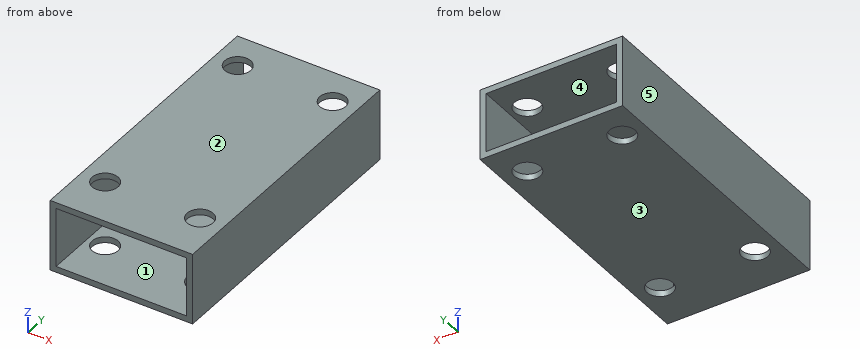
from build123d import *

# Parameters (mm, degrees)
SKETCH1_W               = 76.2
SKETCH1_H               = 38.1
EXTRUDE1_DEPTH          = 76.2
SKETCH2_W               = 69.85
SKETCH2_H               = 31.75
EXTRUDE2_DEPTH          = 159.241184589
F_1_2_CLEARANCE_HOLE1_D = 13.89126


with BuildPart() as part:
    # Sketch1 → Extrude1 (new, symmetric)
    with BuildSketch(Plane(origin=(0, 0, 0), x_dir=(1, 0, 0), z_dir=(0, 1, 0))):
        Rectangle(SKETCH1_W, SKETCH1_H)
    extrude(amount=EXTRUDE1_DEPTH, both=True)

    # Sketch2 → Extrude2 (cut, through all)
    with BuildSketch(Plane(origin=(0, 76.2, 0), x_dir=(1, 0, 0), z_dir=(0, 1, 0))):
        Rectangle(SKETCH2_W, SKETCH2_H)
    extrude(amount=-EXTRUDE2_DEPTH, mode=Mode.SUBTRACT)

    # 1/2 Clearance Hole1 (through all)
    with Locations(Plane.XY.offset(19.05)):
        with Locations((25.4, 57.15), (-25.4, 57.15), (-25.4, -50.8), (25.4, -50.8)):
            Hole(F_1_2_CLEARANCE_HOLE1_D / 2)


solid = part.part
Could you check a few things on this model? Use its own coordinates, in mm. Face numbers are marked on the shaded views. A direction names the side the tool comes from. Give positions to 0.01 mm unless a question says otherwise; leave off trailing zeros. Order: outer loops, then holes, each group sorted by start corner. A loop starts at its lowest first (then second) coordinate and runs counter-clockwise, first axis right, second up.
1. Suppose I cut it at D-D (y = 45.5). List the corners of the cut face in (x, z) for me (3 decimals), plus the area to 3 significant figures.
2. For the marked faces 1 and 2, which set-ups out of +Z, -Z, +X, -X, +Y, -Y let a thin tool reach every point of the face, with its end or its side?
3. I need wall thicknesses on L1, parallel to Y at x = -25, z = -17; L2, parallel to X at y = 57, z = 16; L3, parallel to Z at x = 9.5, y = 7.5 (3 decimals). Which ranges of each line are inside material? Lowest first, please.
4. Will this pin go through, and if not, where does the flat tip stop? P1, Ø18, axis at x = -25.4, y = 57.15, coming from the -Z side.
5. Suppose I cut it at A-A (z = -9). List the corners of the cut face in (x, y) for me (3 decimals), plus the area to 3 significant figures.
6. Suppose I cut it at B-B (x = 25.4). List the corners of the cut face in (y, z) for me (3 decimals), plus the area to 3 significant figures.
7. We'd pull the mould along Z, two halves only. Please class the marked faces 3, 4 and 5: pulls with the +Z half, pulls with the -Z half, needs draft (parallel to the pull), parting line crosses it, or undercut.
8. Suppose I cut it at C-C (y = -47.5). List the corners of the cut face in (x, z) for me (3 decimals), plus the area to 3 significant figures.
Solved:
1. outline: (-38.1, -19.05) - (38.1, -19.05) - (38.1, 19.05) - (-38.1, 19.05) - close; hole (-34.925, -15.875) - (34.925, -15.875) - (34.925, 15.875) - (-34.925, 15.875) - close
1. area: 685 mm2
2. face 1: +Y, -Y
2. face 2: +Z, +X, -X, +Y, -Y
3. L1: y = -76.2 to -57.73, -43.87 to 50.22, 64.08 to 76.2
3. L2: x = -38.1 to -32.34, -18.46 to 18.46, 32.34 to 38.1
3. L3: z = -19.05 to -15.875, 15.875 to 19.05
4. P1: stops at z = -19.05
5. outline: (-38.1, -76.2) - (-34.925, -76.2) - (-34.925, 76.2) - (-38.1, 76.2) - close; (34.925, -76.2) - (38.1, -76.2) - (38.1, 76.2) - (34.925, 76.2) - close
5. area: 968 mm2
6. outline: (-76.2, -19.05) - (-57.746, -19.05) - (-57.746, -15.875) - (-76.2, -15.875) - close; (-76.2, 15.875) - (-57.746, 15.875) - (-57.746, 19.05) - (-76.2, 19.05) - close; (-43.854, -19.05) - (50.204, -19.05) - (50.204, -15.875) - (-43.854, -15.875) - close; (-43.854, 15.875) - (50.204, 15.875) - (50.204, 19.05) - (-43.854, 19.05) - close; (64.096, -19.05) - (76.2, -19.05) - (76.2, -15.875) - (64.096, -15.875) - close; (64.096, 15.875) - (76.2, 15.875) - (76.2, 19.05) - (64.096, 19.05) - close
6. area: 791 mm2
7. face 3: pulls with the -Z half
7. face 4: undercut
7. face 5: needs draft
8. outline: (-38.1, -19.05) - (-31.512, -19.05) - (-31.512, -15.875) - (-34.925, -15.875) - (-34.925, 15.875) - (-31.512, 15.875) - (-31.512, 19.05) - (-38.1, 19.05) - close; (-19.288, -19.05) - (19.288, -19.05) - (19.288, -15.875) - (-19.288, -15.875) - close; (-19.288, 15.875) - (19.288, 15.875) - (19.288, 19.05) - (-19.288, 19.05) - close; (31.512, -19.05) - (38.1, -19.05) - (38.1, 19.05) - (31.512, 19.05) - (31.512, 15.875) - (34.925, 15.875) - (34.925, -15.875) - (31.512, -15.875) - close
8. area: 530 mm2
